Geometry: final body of the model. Coordinates: model frame, mm. A direction names the side the tool comes from. Give positions to 0.01 mm unless a question says otherwise; leave off trailing zeros. Order: outer loops, then holes, each group sorted by start corner. A loop starts at its lowest first (then second) coordinate and runs counter-clockwise, first axis right, second up. Notation, with made-up numbers: (-11.75, 13) -> (28.25, 13) arc R26 ccw to (28.25, 41) -> close; hole circle Ø3 at (30.5, -1.75). An arc over 180 degrees is marked (long way). Answer in a Markdown table with one row per item. Add a question column.
Q1. Cut plane A-A on y = 25.5. Return the cut outline in (x, z), and give its area (3 significant figures).
Q2. Cut plane D-D on z = 37.5. Return the cut outline in (x, y), and give its area (3 significant figures).
Q3. Contact query for flat-ended pins moving along their axis: P1, Ø1.5, axis at x = 58.5, z = 17.5, coming from the +Y side; P2, Ø5, axis at y = 35.5, z = 36, coming from the +X side; P3, Ø12, axis at x = 31, z = 14.5, coming from the +Y side (3 decimals). Output: stop coordinate, or through.
Q4. Cut plane B-B on z = 16. Return the cut outline in (x, y).
Q5. Line query: line 1 along X through (y, z) = (5.75, 20); line 2 along X through (y, z) = (3.5, 26); line 3 along Y through (x, z) = (-58.5, 38). Output: solid intervals per line, ascending. Write a range as from..to.
Q6. Set-up query: faces 5 (the face through (0.649, 39.995, 19.72)), 6 (the face through (67, 10, 20)), 7 (the face through (-32.68, 2.04, 19.72)). Return all of +Z, -Z, +X, -X, +Y, -Y with unobstructed straight access to the full face (end or side cutting, diameter ignored); none if empty.
Q7. Pull-direction query (X, two-part tool) for faces 1 (the face through (40.4, 11.6, 19.7)), 2 (the face through (32.533, 2.151, 19.72)), 3 (the face through (-67, 10, 20)), 4 (the face through (-0.554, 29.995, 19.72)); classes: +X half, -X half, draft (parallel to the pull), parting line (faces both ways), or undercut.
Q8. Cut plane C-C on x = 57. Return the cut outline in (y, z), and give its area (3 significant figures).
from build123d import *

# Parameters (mm, degrees)
BOSS_EXTRUDE1_DEPTH = 40
FILLET1_R           = 20
SKETCH2_R           = 7.5
CUT_EXTRUDE1_DEPTH  = 40


with BuildPart() as part:
    # Sketch1 → Boss-Extrude1 (new body)
    with BuildSketch(Plane.XY):
        with BuildLine():
            Line((-100, 0), (-38.729833462, 0))
            ThreePointArc((-38.729833462, 0), (-32.606109105, 2.09430585), (-29.047375097, 7.5))
            ThreePointArc((-29.047375097, 7.5), (0, 30), (29.047375097, 7.5))
            ThreePointArc((29.047375097, 7.5), (32.606109105, 2.09430585), (38.729833462, 0))
            Line((38.729833462, 0), (100, 0))
            Line((100, 0), (100, 10))
            Line((100, 10), (45.82575695, 10))
            ThreePointArc((45.82575695, 10), (40.348531375, 11.633399735), (36.66060556, 16))
            ThreePointArc((36.66060556, 16), (0, 40), (-36.66060556, 16))
            ThreePointArc((-36.66060556, 16), (-40.348531375, 11.633399735), (-45.82575695, 10))
            Line((-45.82575695, 10), (-100, 10))
            Line((-100, 10), (-100, 0))
        make_face()
    extrude(amount=BOSS_EXTRUDE1_DEPTH)

    # Fillet1
    fillet1_edges = [part.edges().sort_by_distance(p)[0] for p in [
        (100, 5, 0),
        (100, 5, 40),
        (-100, 5, 0),
        (-100, 5, 40),
    ]]
    fillet(fillet1_edges, radius=FILLET1_R - 0.0001)  # a hair under: the kernel refuses the full size

    # Sketch2 → Cut-Extrude1 (cut)
    with BuildSketch(Plane(origin=(0, 10, 0), x_dir=(1, 0, 0), z_dir=(0, 1, 0))):
        with Locations(Location((-80, -20, 0), (0, 0, 270))):
            Circle(SKETCH2_R)
        with Locations(Location((80, -20, 0), (0, 0, 270))):
            Circle(SKETCH2_R)
    extrude(amount=-CUT_EXTRUDE1_DEPTH, mode=Mode.SUBTRACT)


solid = part.part
Completed:
| question | item | result |
|---|---|---|
| 1 | outline | (-30.82, 0) -> (-15.8, 0) -> (-15.8, 40) -> (-30.82, 40) -> close; (15.8, 0) -> (30.82, 0) -> (30.82, 40) -> (15.8, 40) -> close |
| 1 | area | 1,200 mm² |
| 2 | outline | (-89.68, 0) -> (-38.73, 0) arc R10 ccw to (-29.05, 7.5) arc R30 cw to (29.05, 7.5) arc R10 ccw to (38.73, 0) -> (89.68, 0) -> (89.68, 10) -> (45.83, 10) arc R10 cw to (36.66, 16) arc R40 ccw to (-36.66, 16) arc R10 cw to (-45.83, 10) -> (-89.68, 10) -> close |
| 2 | area | 2,090 mm² |
| 3 | P1 | stops at y = 10 |
| 3 | P2 | stops at x = 22.61 |
| 3 | P3 | stops at y = 31.225 |
| 4 | outline | (-99.6, 0) -> (-86.34, 0) -> (-86.34, 10) -> (-99.6, 10) -> close; (-73.66, 0) -> (-38.73, 0) arc R10 ccw to (-29.05, 7.5) arc R30 cw to (29.05, 7.5) arc R10 ccw to (38.73, 0) -> (73.66, 0) -> (73.66, 10) -> (45.83, 10) arc R10 cw to (36.66, 16) arc R40 ccw to (-36.66, 16) arc R10 cw to (-45.83, 10) -> (-73.66, 10) -> close; (86.34, 0) -> (99.6, 0) -> (99.6, 10) -> (86.34, 10) -> close |
| 5 | line 1 | x = -100..-87.5, -72.5..-29.68, 29.68..72.5, 87.5..100 |
| 5 | line 2 | x = -99.08..-84.5, -75.5..-31.13, 31.13..75.5, 84.5..99.08 |
| 5 | line 3 | y = 0..10 |
| 6 | face 5 | +Z, -Z, +Y |
| 6 | face 6 | +Z, -Z, +X, +Y |
| 6 | face 7 | +Z, -Z, -Y |
| 7 | face 1 | +X half |
| 7 | face 2 | undercut |
| 7 | face 3 | draft |
| 7 | face 4 | undercut |
| 8 | outline | (0, 0) -> (10, 0) -> (10, 40) -> (0, 40) -> close |
| 8 | area | 400 mm² |
